Autodesk Inventor part; units mm, degrees
ref_plane "Płaszczyzna konstrukcyjna1" through (-22.5, -96.5, -27.5684) normal (0, 0, -1) x (0, 1, 0)
ref_plane "YZ Plane" through (0, 0, 0) normal (1, 0, 0) x (0, 1, 0)
ref_plane "XZ Plane" through (0, 0, 0) normal (0, 1, 0) x (-1, 0, 0)
sketch "Szkic1" plane through (0, 0, 0) normal (0, 0, 1) x (1, 0, 0)
  line L0 (16, -77.5) -> (-16, -77.5)
  line L1 (-16, -77.5) -> (-16, -96.5)
  line L2 (-16, -96.5) -> (16, -96.5)
  line L3 (16, -96.5) -> (16, -77.5)
  point P0 (0, 0)
  dimension "d1" = 32
extrude "Wyciągnięcie proste1" add sketch "Szkic1" against normal blind 1.5
sketch "Szkic2" plane through (0, 0, -1.5) normal (0, 0, -1) x (-1, 0, 0)
  line L0 (-16, -77.5) -> (-16, -96.5)
  line L1 (16, -96.5) -> (-16, -96.5)
  line L2 (-16, -96.5) -> (-16, -95)
  line L3 (-16, -95) -> (16, -95)
  line L4 (16, -95) -> (16, -96.5)
  point P0 (0, 0)
  dimension "d5" = 1.5
ref_plane "Płaszczyzna konstrukcyjna1" through (-22.5, -96.5, -27.5684) normal (0, 0, -1) x (0, 1, 0)
extrude "Wyciągnięcie proste2" add sketch "Szkic2" along normal up to surface (26.0684 mm away)
fillet "Zaokrąglenie1" radius 1 1 edges at (0, -96.5, 0)
properties part number "ZAŚLEPKA PRZEDNIA DOLNA CZARNEJ OBUDOWY STOJAKA" material "Tworzywo sztuczne, nieprzezroczyste czarne"
Source: CAD feature listing. Evaluate the final solid. Frame: model axes, mm. A direction names the side the tool comes from. Give positions to 0.01 mm unless a question says otherwise; leave off trailing zeros. Write each loop counter-clockwise with the first axis right and the second up, starting at its lowest first coordinate (ties: lowest second). Pieces come first, ordered by that corner, then holes. Notation, with made-up numbers: (27.5, 38) -> (32.5, 38) arc R4 ccw to (32.5, 42) -> close; hole circle Ø8 at (12.5, -27). An arc over 180 degrees is marked (long way). Return JSON: item names as keys, results as strings. Group by question number.
1. Section B-B, the plane y = -86.25. Output: boundary loops of the cut face in (x, z).
2. Material intervals for line 1 (Z direction, x = 14, y = -93.75); line 2 (Y direction, x = -8.5, z = -4.5), sorted ascending. Write a range as from..to.
3. Pin query (flat end, axial travel): pin 1 Ø9 at (x, y) = (-4.5, -89.5) entering from -Z; pin 2 Ø5 at (x, y) = (-7.5, -82) entering from +Z; pin 3 Ø4 at (x, z) = (-9.5, -10) entering from +Y. Return the tip coordinate at first contact, or that it passes through.
4. Access query for faces 1 (the face through (0, -86, -1.5)), 2 (the face through (16, -95.5, -7.6)). Directions: +Z, -Z, +X, -X, +Y, -Y. A direction counts if a zero-diameter tool reaches every point of the face in a straight line with its end or side. Return the directions, or none.
5. Section C-C, the plane z = -8.25. Output: boundary loops of the cut face in (x, y).
6. Section A-A, the plane x = 0. Output: boundary loops of the cut face in (y, z).
Determined:
{
 "1": {"outline": "(-16, -1.5) -> (16, -1.5) -> (16, 0) -> (-16, 0) -> close"},
 "2": {"line 1": "z = -1.5..0", "line 2": "y = -96.5..-95"},
 "3": {"pin 1": "stops at z = -1.5", "pin 2": "stops at z = 0", "pin 3": "stops at y = -95"},
 "4": {"face 1": "-Z, +X, -X, +Y", "face 2": "+Z, -Z, +X, +Y, -Y"},
 "5": {"outline": "(-16, -96.5) -> (16, -96.5) -> (16, -95) -> (-16, -95) -> close"},
 "6": {"outline": "(-96.5, -27.57) -> (-95, -27.57) -> (-95, -1.5) -> (-77.5, -1.5) -> (-77.5, 0) -> (-95.5, 0) arc R1 ccw to (-96.5, -1) -> close"}
}
